```python
from build123d import *

# Parameters (mm, degrees)
EXTRUDE_1_DEPTH           = 5
HOLE_WIZARD_1_D           = 3.2
HOLE_WIZARD_1_DEPTH       = 10
HOLE_WIZARD_1_CBORE_D     = 6
HOLE_WIZARD_1_CBORE_DEPTH = 3.4
HOLE_WIZARD_M3_1_D        = 2.5
SKETCH_9_W                = 15
SKETCH_9_H                = 10
EXTRUDE_2_DEPTH           = 1
HOLE_WIZARD_M4_1_D        = 3.3
HOLE_WIZARD_M4_1_DEPTH    = 9.5
HOLE_WIZARD_M4_1_TIP      = 0.991420021


with BuildPart() as part:
    # 草图1 → 凸台-拉伸1 (new, symmetric)
    with BuildSketch(Plane(origin=(0, 0, 0), x_dir=(1, 0, 0), z_dir=(0, 1, 0))):
        with BuildLine():
            Line((11, -15), (-11, -15))
            Line((-11, -15), (-11, 15))
            Line((-11, 15), (-1, 15))
            Line((-1, 15), (-1, 7.937253933))
            ThreePointArc((-1, 7.937253933), (0, -8), (1, 7.937253933))
            Line((1, 7.937253933), (1, 15))
            Line((1, 15), (11, 15))
            Line((11, 15), (11, -15))
        make_face()
    extrude(amount=EXTRUDE_1_DEPTH, both=True)

    # 打孔尺寸(%根据)内六角圆柱头螺钉的类型1
    with Locations(Plane(origin=(11, 0, 0), x_dir=(0, 0, -1), z_dir=(1, 0, 0))):
        with Locations((11, 0)):
            CounterBoreHole(HOLE_WIZARD_1_D / 2, HOLE_WIZARD_1_CBORE_D / 2, HOLE_WIZARD_1_CBORE_DEPTH, depth=HOLE_WIZARD_1_DEPTH)

    # M3 螺纹孔1 (through all)
    with Locations(Plane.ZY.offset(11)):
        with Locations((-11, 0)):
            Hole(HOLE_WIZARD_M3_1_D / 2)

    # 草图9 → 凸台-拉伸2 (add)
    with BuildSketch(Plane(origin=(11, 0, 0), x_dir=(0, 0, -1), z_dir=(1, 0, 0))):
        with Locations((-7.5, 0)):
            Rectangle(SKETCH_9_W, SKETCH_9_H)
    extrude(amount=EXTRUDE_2_DEPTH)

    # M4 螺纹孔1
    with Locations(Plane(origin=(12, 0, 7), x_dir=(0, 0, 1), z_dir=(1, 0, 0))):
        with Locations((3, 0)):
            Hole(HOLE_WIZARD_M4_1_D / 2, depth=HOLE_WIZARD_M4_1_DEPTH)
            with Locations((0, 0, -(HOLE_WIZARD_M4_1_DEPTH + HOLE_WIZARD_M4_1_TIP / 2))):  # 118° drill point
                Cone(0, HOLE_WIZARD_M4_1_D / 2, HOLE_WIZARD_M4_1_TIP, mode=Mode.SUBTRACT)


solid = part.part
```
The model under review builds one solid part; all positions refer to its coordinate system, in mm. A direction names the side the tool comes from. Round coordinates to 2 decimals unless told otherwise and drop trailing zeros. Loops run counter-clockwise (first coordinate to the right, second up) from the corner with the lowest first, then second, coordinate; pieces in that order, holes last. Notation, with made-up numbers: (49, 42) - (100, 42) arc R31 ccw to (100, 72) - close; hole circle Ø5 at (82, -28). An arc over 180 degrees is marked (long way). Write each question's results on one line, items separated by ' | '. Start each with the question number.
Q1. Take a section at B-B on z = -11. Give the boundary of the cut face in (x, y).
Q2. Take a section at A-A on x = -7. Give the boundary of the cut face in (y, z).
Q3. Wall thickness on line 1 along Y through (x, z) = (-3.25, -10.25); line 2 along Y through (x, z) = (10.25, 10); line 3 along X through (y, z) = (0, -8.25): over which ranges is each line inside the solid? List them lowest first. Write a range as [from, to].
Q4. Take a section at C-C on z = 7.25. Give the boundary of the cut face in (x, y), plus the area to 3 significant figures.
Q5. Draft analysis for pull direction X (two halves, no side actions). For faces 6 (the cylindrical face through (4.25, 0.07, -12.6)), 7 (the conical face through (1.7, 0.1, 10.3)), 8 (the cylindrical face through (0, 0, 8)), state which applies: pulls with the +X half, pulls with the -X half, needs draft (parallel to the pull), parting line crosses it, or undercut.
Q6. Insertion check: P1, Ø2, axis at y = 0, z = -11, coming from the +X side. The pin has a flat end and moves straight along its axis. Give the tip position at first contact, or say it passes through.
Q7. Tool access review of faces 1 (the flat face through (-1, 1, -12)), 2 (the flat face through (-11, 0, 0)), 3 (the flat face through (11, 0.1, -7.6)), 4 (the cylindrical face through (9.3, -1.8, -8.6)), 5 (the flat face through (-6, 0, -15)): name each direction out of +Z, -Z, +X, -X, +Y, -Y from which nothing blocks a thin tool from reaching the whole face with its end or side.
Q8. Take a section at D-D on y = 0.5. Give the number of separate pieces and of enclosed holes in the cut face, plus the area to 3 significant figures.
Data:
1) outline: (-11, -5) - (-1, -5) - (-1, -1.25) - (-11, -1.25) - close; (-11, 1.25) - (-1, 1.25) - (-1, 5) - (-11, 5) - close; (1, -5) - (11, -5) - (11, -3) - (7.6, -3) - (7.6, -1.6) - (1, -1.6) - close; (1, 1.6) - (7.6, 1.6) - (7.6, 3) - (11, 3) - (11, 5) - (1, 5) - close
2) outline: (-5, -15) - (5, -15) - (5, -3.87) - (-5, -3.87) - close; (-5, 3.87) - (5, 3.87) - (5, 15) - (-5, 15) - close; hole circle Ø2.5 at (0, -11)
3) line 1: y = [-5, -1], [1, 5] | line 2: y = [-5, -1.65], [1.65, 5] | line 3: x = [-11, -1], [1, 7.6]
4) outline: (-11, -5) - (-3.38, -5) - (-3.38, 5) - (-11, 5) - close; (3.38, -5) - (12, -5) - (12, 5) - (3.38, 5) - close | area: 162 mm²
5) face 6: needs draft | face 7: pulls with the +X half | face 8: undercut
6) P1: passes through
7) face 1: -Z, +Y, -Y | face 2: +Z, -Z, -X, +Y, -Y | face 3: -Z, +X, +Y, -Y | face 4: +X | face 5: -Z, +X, -X, +Y, -Y
8) separate pieces: 3 | enclosed holes: 0 | area: 366 mm²
